```python
from build123d import *

# Parameters (mm, degrees)
SKETCH1_R           = 22.225
SKETCH1_R_2         = 4.7625
BOSS_EXTRUDE1_DEPTH = 95.25
SKETCH2_R           = 12.7
BOSS_EXTRUDE2_DEPTH = 38.1
BOSS_EXTRUDE3_START = -10.16
BOSS_EXTRUDE3_DEPTH = 101.6
CUT_EXTRUDE1_DEPTH  = 6.35
SKETCH5_R           = 3.175
BOSS_EXTRUDE4_DEPTH = 6.35
DOME1_FACE_RADIUS   = 3.175
DOME1_HEIGHT        = 25.4


with BuildPart() as part:
    # Sketch1 → Boss-Extrude1 (new body)
    with BuildSketch(Plane(origin=(0, 0, 0), x_dir=(1, 0, 0), z_dir=(0, 1, 0))):
        with Locations(Location((0, 0, 0), (0, 0, 270))):
            Circle(SKETCH1_R)
        with Locations(Location((0, 0, 0), (0, 0, 270))):
            Circle(SKETCH1_R_2, mode=Mode.SUBTRACT)
    extrude(amount=BOSS_EXTRUDE1_DEPTH)

    # Sketch2 → Boss-Extrude2 (add)
    with BuildSketch(Plane(origin=(0, 0, 0), x_dir=(0, 0, -1), z_dir=(1, 0, 0))):
        with Locations(Location((0, 44.45, 0), (0, 0, 180))):
            Circle(SKETCH2_R)
    extrude(amount=BOSS_EXTRUDE2_DEPTH)

    # Sketch3 → Boss-Extrude3 (add)
    with BuildSketch(Plane(origin=(0, 0, 0), x_dir=(0, 0, -1), z_dir=(1, 0, 0)).offset(BOSS_EXTRUDE3_START)):
        Polygon((-34.433625962, 31.155054448), (-31.75, 25.4), (186.942069012, 127.377786558), (184.25844305, 133.132841006), align=None)
    extrude(amount=-BOSS_EXTRUDE3_DEPTH)

    # Sketch4 → Cut-Extrude1 (cut)
    with BuildSketch(Plane(origin=(0, 38.779412625, 18.083137086), x_dir=(1, 0, 0), z_dir=(0, 0.9063077870366493, 0.42261826174070105))):
        with BuildLine():
            Line((-41.964599748, -16.344444393), (-81.980400092, 77.043433422))
            Line((-81.980400092, 77.043433422), (-81.980400092, 223.25923161))
            Line((-81.980400092, 223.25923161), (-111.76, 223.25923161))
            Line((-111.76, 223.25923161), (-111.76, -18.04076839))
            Line((-111.76, -18.04076839), (-10.16, -18.04076839))
            Line((-10.16, -18.04076839), (-10.16, -1.857678602))
            add(Edge.make_bspline(
                [(-15.398693032, 2.269861536), (-13.053103619, -0.216913648), (-10.16, -1.857678602)],
                knots=[5.477258717, 5.477258717, 5.477258717, 5.808405234, 5.808405234, 5.808405234], degree=2, weights=[0.860760797, 0.917991521, 1]))
            Line((-15.398693032, 2.269861536), (-12.78088793, -3.839506786))
            Line((-12.78088793, -3.839506786), (-41.964599748, -16.344444393))
        make_face()
        with BuildLine():
            Line((-10.16, 223.25923161), (-50.230400092, 223.25923161))
            Line((-50.230400092, 223.25923161), (-50.230400092, 83.55923161))
            Line((-50.230400092, 83.55923161), (-22.157554012, 18.043522888))
            add(Edge.make_bspline(
                [(-10.16, 41.762746934), (-23.308412463, 34.30589187), (-22.157554012, 18.043522888)],
                knots=[3.616372727, 3.616372727, 3.616372727, 4.782388845, 4.782388845, 4.782388845], degree=2, weights=[1, 0.711235953, 0.729678603]))
            Line((-10.16, 41.762746934), (-10.16, 223.25923161))
        make_face()
    extrude(amount=-CUT_EXTRUDE1_DEPTH, mode=Mode.SUBTRACT)

    # Sketch5 → Boss-Extrude4 (add)
    with BuildSketch(Plane(origin=(0, 38.779412625, 18.083137086), x_dir=(1, 0, 0), z_dir=(0, 0.906307787036649, 0.4226182617407014))):
        with Locations(Location((-66.105400092, 213.73423161, 0), (0, 0, 270))):
            Circle(SKETCH5_R)
    extrude(amount=BOSS_EXTRUDE4_DEPTH)

    # Dome1: a dome of height H over a round flat face of radius A is a cap of a sphere of radius (A * A + H * H) / (2 * H)
    dome1_r = (DOME1_FACE_RADIUS * DOME1_FACE_RADIUS + DOME1_HEIGHT * DOME1_HEIGHT) / (2 * DOME1_HEIGHT)
    dome1_base = Plane((-66.105400092, 134.86245651, -172.942235416), z_dir=(0, 0.906307787037, 0.422618261741))
    with Locations(dome1_base.offset(DOME1_HEIGHT - dome1_r)):
        dome1_ball = Sphere(dome1_r, mode=Mode.PRIVATE)
    add(split(dome1_ball, bisect_by=dome1_base, keep=Keep.TOP, mode=Mode.PRIVATE))


solid = part.part
```
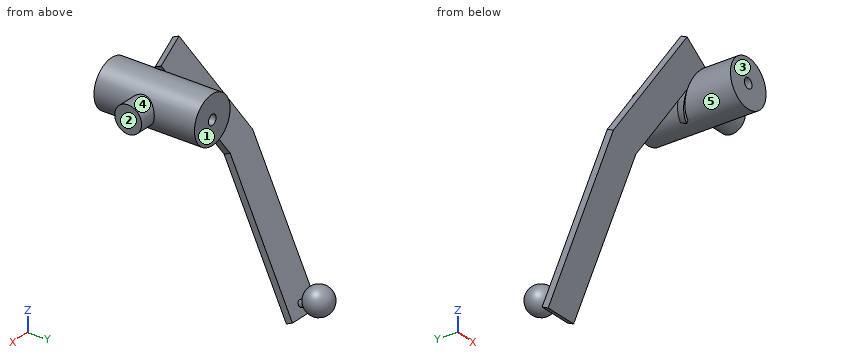
Here's how the part is built. I have some questions about the finished solid (model axes, mm). Face numbers are marked on the shaded views. A direction names the side the tool comes from. Give positions to 0.01 mm unless a question says otherwise; leave off trailing zeros. Write each loop counter-clockwise with the first axis right and the second up, starting at its lowest first coordinate (ties: lowest second). Pieces come first, ordered by that corner, then holes. Notation, with made-up numbers: M 46,23 L 86,23 A26 cw 86,44 Z; hole C 68,85.25 d7. An arc over 180 degrees is marked long. Put each result on its own line as item: value. Start each with the question number.
Item 1: If we section it at D-D, the plane y = 110: Write out the boundary of the cut face in (x, z).
Item 2: On a 3-axis mill with a long thin cutter (end or side, diameter ignored), from which of +Z, -Z, +X, -X, +Y, -Y can I reach the whole of each face in a straight line? I mean the marked faces 3, 4 and 5. Say none if no direction works.
Item 3: Will these pins go through, and if not, where does the flat tip stop? pin 1 (1.5 mm diameter, centred on x = -65, y = 138.5, fed in from -Z); pin 2 (3 mm diameter, centred on y = 33, z = 19, fed in from -X); pin 3 (12 mm diameter, centred on x = -22, y = 86, fed in from +Z).
Item 4: If we section it at C-C, the plane z = -117: Write out the boundary of the cut face in (x, y).
Item 5: Thinking about a two-plate mould opening in X: for the marked faces 1 and 2, which applies, +X half, -X half, draft (parallel to the pull), parting line (faces both ways), or undercut?
Item 6: I need wall thicknesses on L1, parallel to X at y = 54.5, z = 0 (1 decimal); L2, parallel to X at y = 23, z = 0 (1 decimal); L3, parallel to Y at x = 18, z = -12.5. Which ranges of each line are inside material? Lowest first, please. Write a range as from..to.
Item 7: If we section it at B-B, the plane x = 26.5: Write out the boundary of the cut face in (y, z), then the cut area to 3 significant figures.
Item 8: If we section it at A-A, the plane y = 82: Count the separate pieces of the cut face and the enclosed holes in it, then the cut area to 3 significant figures.
Values:
1. outline: M -81.98,-149.68 L -50.23,-149.68 L -50.23,-134.65 L -81.98,-134.65 Z
2. face 3: +Z, -Z, +X, -X, -Y
2. face 4: +X
2. face 5: none
3. pin 1: z = -178.48
3. pin 2: x = -48.21
3. pin 3: z = 15.43
4. outline: M -81.98,94.76 L -50.23,94.76 L -50.23,101.77 L -81.98,101.77 Z
5. face 1: draft
5. face 2: +X half
6. L1: -22.2..-4.8, 0..38.1
6. L2: -22.2..-4.8, 4.8..22.2
6. L3: 0..95.25
7. outline: C 44.45,0 d25.4
7. area: 507 mm²
8. separate pieces: 2
8. enclosed holes: 1
8. area: 1,960 mm²
